Here's how the part is built. I have some questions about the finished solid (model axes, mm). A direction names the side the tool comes from. Give positions to 0.01 mm unless a question says otherwise; leave off trailing zeros. Loops run counter-clockwise (first coordinate to the right, second up) from the corner with the lowest first, then second, coordinate; pieces in that order, holes last.
Q1. Thinking about a two-plate mould opening in X: for faces 3 (the face through (26, 15, 6.312)), 4 (the face through (17.535, 33.713, 9.86)), 5 (the face through (16, -16, 0)), which applies, pulls with the +X half, pulls with the -X half, needs draft (parallel to the pull), parting line crosses it, or undercut?
Q2. Suppose I cut it at A-A (y = 0). List the corners of the cut face in (x, z) for me.
Q3. I need wall thicknesses on probe 1 along Y at (x, z) = (0, 12.5); probe 2 along X at (y, z) = (17.5, 5.5); probe 3 along Y at (x, z) = (2, 10.5). Which ranges of each line are inside material? Lowest first, please.
Q4. Suppose I cut it at B-B (x = 12.5). List the corners of the cut face in (y, z) for me, and give its area (3 significant figures).
Q5. I'm going to push flat-ended pins straight in: P1, Ø10, axis at x = 7, z = 16.5, coming from the -Y side; P2, Ø3, axis at y = 4, z = 10.5, coming from the +X side; P3, Ø2.5, axis at x = 0.5, y = -30.5, coming from the -Z side. Where does each tip first touch, or does it pass through?
Q6. Suppose I cut it at D-D (z = 2.25). List the corners of the cut face in (x, y) for me, and give its area (3 significant figures).
Q7. For faces 1 (the face through (-4.769, 21.477, 9.86)), 2 (the face through (-26, 15, 6.312)), which set-ups out of +Z, -Z, +X, -X, +Y, -Y let a thin tool reach every point of the face, with its end or its side?
Q8. Suppose I cut it at C-C (z = 11). List the corners of the cut face in (x, y) for me, and give its area (3 significant figures).
Autodesk Fusion 360 part; units mm, degrees
sketch "Sketch1" plane through (0, 0, 0) normal (0, 0, 1) x (1, 0, 0)
  circle A0 centre (0, 0) radius 19.3
  circle A1 centre (0, 0) radius 22.5
  circle A2 centre (0, 0) radius 38
  dimension "d1" = 45
  dimension "d2" = 38.6
  dimension "d3" = 76
extrude "Extrude1" add sketch "Sketch1" along normal blind 20 contours A1
sketch "Sketch2" plane through (0, 0, 0) normal (0, 0, 1) x (1, 0, 0)
  circle A0 centre (0.2654, -30.1553) radius 2.5
  dimension "d8" = 5
extrude "Extrude4" add sketch "Sketch1" along normal blind 20 contours A1 | A2
extrude "Extrude5" cut sketch "Sketch2" along normal blind 6.312
pattern_circular "C-Pattern2" count 3 over 360 about axis through (0, 0, 20) along (0, 0, 1) of "Extrude5"
move_face "면 간격띄우기1" offset 5 1 faces at (19.276, -0.962, 13.3333)
move_face "면 간격띄우기2" offset 2.3 1 faces at (14.2822, 0.7128, 6.6667)
move_face "면 간격띄우기3" offset -10 1 faces at (11.9851, 0.5982, 6.6667)
Solutions:
1. face 3: undercut
1. face 4: parting line crosses it
1. face 5: needs draft
2. outline: (-38, 0) - (-22, 0) - (-22, 20) - (-38, 20) - close; (22, 0) - (38, 0) - (38, 20) - (22, 20) - close
3. probe 1: y = -38 to -22, 22 to 38
3. probe 2: x = -33.73 to -13.33, 13.33 to 24.78, 27.18 to 33.73
3. probe 3: y = -37.95 to -21.91, 21.91 to 37.95
4. outline: (-35.89, 0) - (-18.1, 0) - (-18.1, 20) - (-35.89, 20) - close; (18.1, 0) - (35.89, 0) - (35.89, 20) - (18.1, 20) - close
4. area: 711 mm2
5. P1: stops at y = -37.95
5. P2: stops at x = 37.92
5. P3: stops at z = 6.31
6. outline: circle Ø76 at (0, 0); hole circle Ø5 at (-26.25, 14.85); hole circle Ø44 at (0, 0); hole circle Ø5 at (0.27, -30.16); hole circle Ø5 at (25.98, 15.31)
6. area: 2,960 mm2
7. face 1: +Z, -Z
7. face 2: -Z
8. outline: circle Ø76 at (0, 0); hole circle Ø44 at (0, 0)
8. area: 3,020 mm2
